```python
from build123d import *

# Parameters (mm, degrees)
SKETCH1_W                                      = 38
SKETCH1_H                                      = 27
EXTRUDE1_DEPTH                                 = 20
SKETCH2_R                                      = 11
LIGHT_WEIGHTING_HOLE_DEPTH                     = 21
LIGHT_WEIGHTING_HOLE_DEPTH_BACK                = 21
F_4_40_TAPPED_HOLE1_D                          = 2.2606
F_4_40_TAPPED_HOLE1_DEPTH                      = 8.8646
F_4_40_TAPPED_HOLE1_TIP                        = 0.679152758
CBORE_FOR_8_SOCKET_HEAD_CAP_SCREW1_D           = 4.3053
CBORE_FOR_8_SOCKET_HEAD_CAP_SCREW1_CBORE_D     = 7.9375
CBORE_FOR_8_SOCKET_HEAD_CAP_SCREW1_CBORE_DEPTH = 4.1656
SKETCH9_W                                      = 0.25
SKETCH9_H                                      = 4
SKETCH9_W_2                                    = 2.002359623
SKETCH9_H_2                                    = 0.25
SKETCH9_W_3                                    = 2.12486514
CUT_EXTRUDE1_DEPTH                             = 0.25


with BuildPart() as part:
    # Sketch1 → Extrude1 (new body, symmetric)
    with BuildSketch(Plane.XY):
        with Locations((0, 13.5)):
            Rectangle(SKETCH1_W, SKETCH1_H)
    extrude(amount=EXTRUDE1_DEPTH, both=True)

    # Sketch2 → Light-Weighting Hole (cut, two sides)
    with BuildSketch(Plane.XY) as light_weighting_hole_sk:
        with Locations((0, 14.5)):
            Circle(SKETCH2_R)
    extrude(amount=LIGHT_WEIGHTING_HOLE_DEPTH, mode=Mode.SUBTRACT)
    extrude(light_weighting_hole_sk.sketch, amount=-LIGHT_WEIGHTING_HOLE_DEPTH_BACK, mode=Mode.SUBTRACT)

    # #4-40 Tapped Hole1
    with Locations(Plane(origin=(0, 27, 0), x_dir=(-1, 0, 0), z_dir=(0, 1, 0))):
        with Locations((13, -16), (13, 16)):
            Hole(F_4_40_TAPPED_HOLE1_D / 2, depth=F_4_40_TAPPED_HOLE1_DEPTH)
            with Locations((0, 0, -(F_4_40_TAPPED_HOLE1_DEPTH + F_4_40_TAPPED_HOLE1_TIP / 2))):  # 118° drill point
                Cone(0, F_4_40_TAPPED_HOLE1_D / 2, F_4_40_TAPPED_HOLE1_TIP, mode=Mode.SUBTRACT)

    # CBORE for #8 Socket Head Cap Screw1 (through all)
    with Locations(Plane(origin=(0, 27, 0), x_dir=(-1, 0, 0), z_dir=(0, 1, 0))):
        with Locations((13.5, 0), (-13.5, 0)):
            CounterBoreHole(CBORE_FOR_8_SOCKET_HEAD_CAP_SCREW1_D / 2, CBORE_FOR_8_SOCKET_HEAD_CAP_SCREW1_CBORE_D / 2, CBORE_FOR_8_SOCKET_HEAD_CAP_SCREW1_CBORE_DEPTH)

    # Sketch9 → Cut-Extrude1 (cut)
    with BuildSketch(Plane(origin=(0, 27, 0), x_dir=(-1, 0, 0), z_dir=(0, 1, 0))):
        with Locations((13.026450264, -18)):
            Rectangle(SKETCH9_W, SKETCH9_H)
        with Locations((12.998090527, 18)):
            Rectangle(SKETCH9_W, SKETCH9_H)
        with Locations((-17.998820188, 0)):
            Rectangle(SKETCH9_W_2, SKETCH9_H_2)
        with Locations((17.93756743, 0)):
            Rectangle(SKETCH9_W_3, SKETCH9_H_2)
    extrude(amount=-CUT_EXTRUDE1_DEPTH, mode=Mode.SUBTRACT)


solid = part.part
```
For this review, take the finished solid that the model builds, in its own axes (mm). A direction names the side the tool comes from. Give positions to 0.01 mm unless a question says otherwise; leave off trailing zeros. Write each loop counter-clockwise with the first axis right and the second up, starting at its lowest first coordinate (ties: lowest second). Pieces come first, ordered by that corner, then holes. Notation, with made-up numbers: M 41.25,22 L 45.25,22 A19 cw 45.25,35 Z; hole C 19.5,-39 d3. An arc over 180 degrees is marked long. Answer as a JSON object with one key per item and string values. Group by question number.
Item 1: Draft analysis for pull direction Z (two halves, no side actions). For faces 1 (the cylindrical face through (-15.65, 11.26, 0.09)), 2 (the flat face through (0, 2, -20)), 3 (the flat face through (-19, 13, 0)), 4 (the cylindrical face through (-13.897, 22.506, -16.688)), state which applies: +Z half, -Z half, draft (parallel to the pull), parting line (faces both ways), or undercut.
Item 2: Consider section D-D on z = -13.5. Write out the cut boundary in (x, y), plus the area to 3 significant figures.
Item 3: Consider section A-A on y = 14.5. Write out the cut boundary in (x, z).
Item 4: For probe 1 along Z at (x, y) = (13.5, 5); probe 2 along X at (y, z) = (20, 3); probe 3 along Z at (x, y) = (-13, 22.5), list the stretches that pass through material, from the lowest coordinate up. Write a range as [from, to].
Item 5: Consider section B-B on x = 13.5. Write out the cut boundary in (y, z), plus the area to 3 significant figures.
Item 6: Consider section C-C on y = 20.25. Write out the cut boundary in (x, z).
Item 7: Tool access review of faces 5 (the flat face through (12, 22.834, -2)), 6 (the flat face through (0, 2, 20)): name each direction out of +Z, -Z, +X, -X, +Y, -Y from which nothing blocks a thin tool from reaching the whole face with its end or side.
Item 8: For pin 1 Ø2 at (x, y) = (2, 5) entering from -Z; pin 2 Ø7 at (x, z) = (-13.5, 0) entering from +Y, all flat-tipped, find the tip position at first contact; note any pin that passes through.
Check result:
{
 "1": {"face 1": "undercut", "face 2": "-Z half", "face 3": "draft", "face 4": "undercut"},
 "2": {"outline": "M -19,0 L 19,0 L 19,27 L -19,27 Z; hole C 0,14.5 d22", "area": "646 mm^2"},
 "3": {"outline": "M -19,-20 L -11,-20 L -11,20 L -19,20 Z; M 11,-20 L 19,-20 L 19,20 L 11,20 Z; hole C -13.5,0 d4.31; hole C 13.5,0 d4.31"},
 "4": {"probe 1": "z = [-20, -2.15], [2.15, 20]", "probe 2": "x = [-19, -9.53], [9.53, 19]", "probe 3": "z = [-20, -17.13], [-14.87, -2.09], [2.09, 14.87], [17.13, 20]"},
 "5": {"outline": "M 0,-20 L 27,-20 L 27,-3.97 L 22.83,-3.97 L 22.83,-2.15 L 0,-2.15 Z; M 0,2.15 L 22.83,2.15 L 22.83,3.97 L 27,3.97 L 27,20 L 0,20 Z", "area": "949 mm^2"},
 "6": {"outline": "M -19,-20 L -9.38,-20 L -9.38,20 L -19,20 Z; M 9.38,-20 L 19,-20 L 19,20 L 9.38,20 Z; hole C -13.5,0 d4.31; hole C -13,-16 d2.26; hole C -13,16 d2.26; hole C 13.5,0 d4.31"},
 "7": {"face 5": "+Y", "face 6": "+Z, +X, -X, +Y, -Y"},
 "8": {"pin 1": "passes through", "pin 2": "stops at y = 22.83"}
}
